Part model, mm, in its own coordinate system. Round coordinates to 2 decimals unless told otherwise and drop trailing zeros. Order: outer loops, then holes, each group sorted by start corner. A loop starts at its lowest first (then second) coordinate and runs counter-clockwise, first axis right, second up. Notation, with made-up numbers: (-38.75, 64) -> (16.25, 64) arc R21 ccw to (16.25, 80) -> close; hole circle Ø5 at (50, -22). An arc over 180 degrees is marked (long way). Use CSV: the item, a comma, the result in double quotes.
```python
from build123d import *

# Parameters (mm, degrees)
SKETCH1_R           = 1.5
BOSS_EXTRUDE1_DEPTH = 8
SKETCH2_R           = 1.5
CUT_EXTRUDE1_DEPTH  = 10


with BuildPart() as part:
    # Sketch1 → Boss-Extrude1 (new body)
    with BuildSketch(Plane.XY):
        with BuildLine():
            Line((75, -4), (-75, -4))
            ThreePointArc((-75, -4), (-79, 0), (-75, 4))
            Line((-75, 4), (75, 4))
            ThreePointArc((75, 4), (79, 0), (75, -4))
        make_face()
        with Locations((-75, 0)):
            Circle(SKETCH1_R, mode=Mode.SUBTRACT)
        with Locations((75, 0)):
            Circle(SKETCH1_R, mode=Mode.SUBTRACT)
    extrude(amount=BOSS_EXTRUDE1_DEPTH)

    # Sketch2 → Cut-Extrude1 (cut)
    with BuildSketch(Plane.XY.offset(8)):
        Circle(SKETCH2_R)
    extrude(amount=-CUT_EXTRUDE1_DEPTH, mode=Mode.SUBTRACT)


solid = part.part
```
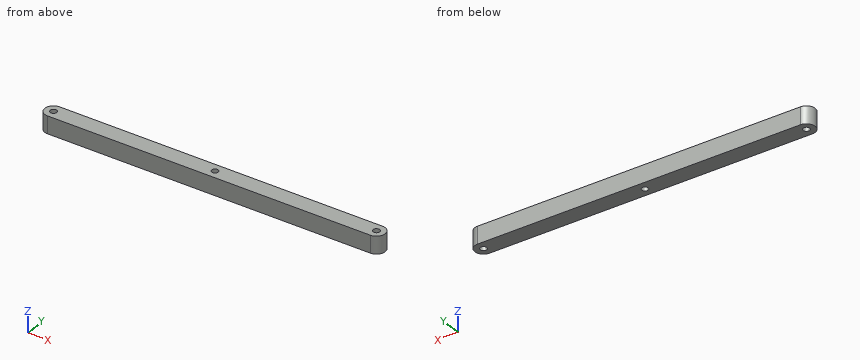
(1) Cut at C-C, the plane x = 0. Give the cut face in (y, z), then the cut area to 3 significant figures.
Reply:
outline,"(-4, 0) -> (-1.5, 0) -> (-1.5, 8) -> (-4, 8) -> close; (1.5, 0) -> (4, 0) -> (4, 8) -> (1.5, 8) -> close"
area,"40.0 mm2"
(2) Cut at B-B, the plane z = 5.5. Give the cut face in (x, y), then the cut area to 3 significant figures.
Reply:
outline,"(-75, -4) -> (75, -4) arc R4 ccw to (75, 4) -> (-75, 4) arc R4 ccw to start; hole circle Ø3 at (-75, 0); hole circle Ø3 at (0, 0); hole circle Ø3 at (75, 0)"
area,"1,230 mm2"
(3) Probe probe 1 along Y at (x, z) = (-75, 5); probe 2 along X at (y, z) = (-0.5, 6); probe 3 along X at (y, z) = (3, 7.75). List the from-to ranges inside material, lowest first. Write a range as [from, to].
Reply:
probe 1,"[-4, -1.5], [1.5, 4]"
probe 2,"[-78.97, -76.41], [-73.59, -1.41], [1.41, 73.59], [76.41, 78.97]"
probe 3,"[-77.65, 77.65]"
(4) Cut at A-A, the plane y = 0. Give the cut face in (x, z).
Reply:
outline,"(-79, 0) -> (-76.5, 0) -> (-76.5, 8) -> (-79, 8) -> close; (-73.5, 0) -> (-1.5, 0) -> (-1.5, 8) -> (-73.5, 8) -> close; (1.5, 0) -> (73.5, 0) -> (73.5, 8) -> (1.5, 8) -> close; (76.5, 0) -> (79, 0) -> (79, 8) -> (76.5, 8) -> close"
